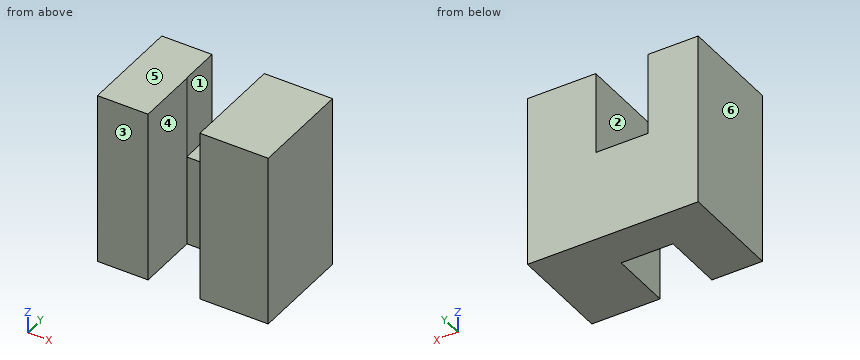
```python
from build123d import *

# Parameters (mm, degrees)
F0_W     = 148.2112929225
F0_H     = 149.8982533813
F1_DEPTH = 144.78
F2_W     = 44.9698530138
F2_H     = 149.8982533813
F3_DEPTH = 109.728
F4_W     = 45.2879443765
F4_H     = 35.052
F5_DEPTH = 71.374
F6_W     = 56.0343910742
F6_H     = 149.8982533813
F7_DEPTH = 158.75


with BuildPart() as f1:
    # F0 (on Front) → F1 (new body)
    with BuildSketch(Plane.XZ):
        with Locations((-14.8211307824, -3.6149062216)):
            Rectangle(F0_W, F0_H)
    extrude(amount=F1_DEPTH)

    # F2 (on face) → F3 (cut)
    with BuildSketch(Plane.XZ.offset(144.78)):
        with Locations((-22.4849265069, -3.6149062216)):
            Rectangle(F2_W, F2_H)
    extrude(amount=-F3_DEPTH, mode=Mode.SUBTRACT)

    # F4 (on face) → F5 (cut)
    with BuildSketch(Plane.XY.offset(71.334220469)):
        with Locations((-22.6439721882, -17.526)):
            Rectangle(F4_W, F4_H)
    extrude(amount=-F5_DEPTH, mode=Mode.SUBTRACT)

    # F6 (on face) → F7 (cut)
    with BuildSketch(Plane.YZ.offset(59.2845156789)):
        with Locations((-116.7628044629, -3.6149062216)):
            Rectangle(F6_W, F6_H)
    extrude(amount=-F7_DEPTH, mode=Mode.SUBTRACT)


solid = f1.part
```
Build history of the part. All positions in model axes, mm. Face numbers are marked on the shaded views. A direction names the side the tool comes from. Coordinates: 2 decimals unless noted, no trailing zeros. Order: outer loops, then holes, each group sorted by start corner. A loop starts at its lowest first (then second) coordinate and runs counter-clockwise, first axis right, second up.
Item 1: Saw through at A-A on z = 38.5. List the corners of the cut face in (x, y), then the cut area to 3 significant figures.
Filled in:
outline: (-88.93, -88.75) - (-44.97, -88.75) - (-44.97, -35.05) - (-45.29, -35.05) - (-45.29, 0) - (-88.93, 0) - close; (0, -88.75) - (59.28, -88.75) - (59.28, 0) - (0, 0) - close
area: 9,150 mm2
Item 2: Tool access for the marked faces 1, 2 and 3: list every direction of +Z, -Z, +X, -X, +Y, -Y with a clear straight run to the whole face (end or side of a thin tool).
Filled in:
face 1: +Z, +Y
face 2: +Z, -Y
face 3: +Z, -Z, +X, -X, -Y
Item 3: Saw through at D-D on x = -26. List the corners of the cut face in (y, z).
Filled in:
outline: (-35.05, -78.56) - (0, -78.56) - (0, -0.04) - (-35.05, -0.04) - close
Item 4: Saw through at B-B on y = -51.5. List the corners of the cut face in (x, z).
Filled in:
outline: (-88.93, -78.56) - (-44.97, -78.56) - (-44.97, 71.33) - (-88.93, 71.33) - close; (0, -78.56) - (59.28, -78.56) - (59.28, 71.33) - (0, 71.33) - close
Item 5: Mould opens along X. For the marked faces 4, 5 and 6 say: released by +X, released by -X, zero draft, split by the parting line, or undercut.
Filled in:
face 4: undercut
face 5: zero draft
face 6: released by -X
Item 6: Drill centre lines: L1, parallel to X at y = -81, z = -59; L2, parallel to Y at x = -41.5, z = -47; L3, parallel to Z at x = -32.5, y = -18.5. Where is each one in solid material? Low to high.
Filled in:
L1: x = -88.93 to -44.97, 0 to 59.28
L2: y = -35.05 to 0
L3: z = -78.56 to -0.04
Item 7: Drop flat-ended pins along their axis: pin 1 Ø13.5 at (x, z) = (-13.5, -41.5) entering from -Y; pin 2 Ø6 at (x, y) = (-0.5, -59) entering from +Z. Give the stop position or say it passes through.
Filled in:
pin 1: stops at y = -35.05
pin 2: stops at z = 71.33
Item 8: Saw through at C-C on z = -14. List the corners of the cut face in (x, y), then the cut area to 3 significant figures.
Filled in:
outline: (-88.93, -88.75) - (-44.97, -88.75) - (-44.97, -35.05) - (0, -35.05) - (0, -88.75) - (59.28, -88.75) - (59.28, 0) - (-88.93, 0) - close
area: 10,700 mm2
